Here's how the part is built. I have some questions about the finished solid (model axes, mm). Give positions to 0.01 mm unless a question says otherwise; leave off trailing zeros. Loops run counter-clockwise (first coordinate to the right, second up) from the corner with the lowest first, then second, coordinate; pieces in that order, holes last.
Q1. Suppose I cut it at B-B (z = 43). List the corners of the cut face in (x, y) for me (3 decimals), and give its area (3 significant figures).
Q2. Suppose I cut it at C-C (x = -1). List the corners of the cut face in (y, z) for me.
Q3. I'm going to push flat-ended pins straight in: P1, Ø3, axis at x = 37.5, z = 31.5, coming from the -Y side (3 decimals); P2, Ø1.6, axis at y = -5, z = 55, coming from the +X side (3 decimals); P3, Ø3, axis at x = -16.5, y = -2.5, coming from the +Z side. Where does each tip first touch, or does it pass through?
Q4. Suppose I cut it at A-A (y = -1). List the corners of the cut face in (x, z) for me (3 decimals), and give its area (3 significant figures).
Q5. I need wall thicknesses on probe 1 along X at (y, z) = (-4.5, 82.5) (3 decimals); probe 2 along X at (y, z) = (-1, 75) (3 decimals); probe 3 along Z at (x, y) = (-15, -3). Which ranges of each line are inside material? Lowest first, please.
```python
from build123d import *

# Parameters (mm, degrees)
F1_DEPTH = 6.35
F2_W     = 6.35
F2_H     = 95.25
F3_DEPTH = 3.175


with BuildPart() as f1:
    # F0 (on Front) → F1 (new body)
    with BuildSketch(Plane.XZ):
        with BuildLine():
            Line((-41.275, 0), (0, 0))
            Line((0, 0), (41.275, 0))
            Line((41.275, 0), (41.275, 95.25))
            Line((41.275, 95.25), (22.225, 95.25))
            Line((22.225, 95.25), (22.225, 73.025))
            ThreePointArc((22.225, 73.025), (21.2950640303, 70.7799359697), (19.05, 69.85))
            Line((19.05, 69.85), (-19.05, 69.85))
            ThreePointArc((-19.05, 69.85), (-21.2950640303, 70.7799359697), (-22.225, 73.025))
            Line((-22.225, 73.025), (-22.225, 95.25))
            Line((-22.225, 95.25), (-41.275, 95.25))
            Line((-41.275, 95.25), (-41.275, 0))
        make_face()
    extrude(amount=F1_DEPTH)

    # F2 (on face) → F3 (cut)
    with BuildSketch(Plane.XZ.offset(6.35)):
        with Locations((-38.1, 47.625)):
            Rectangle(F2_W, F2_H)
        with Locations((38.1, 47.625)):
            Rectangle(F2_W, F2_H)
    extrude(amount=-F3_DEPTH, mode=Mode.SUBTRACT)


solid = f1.part
```
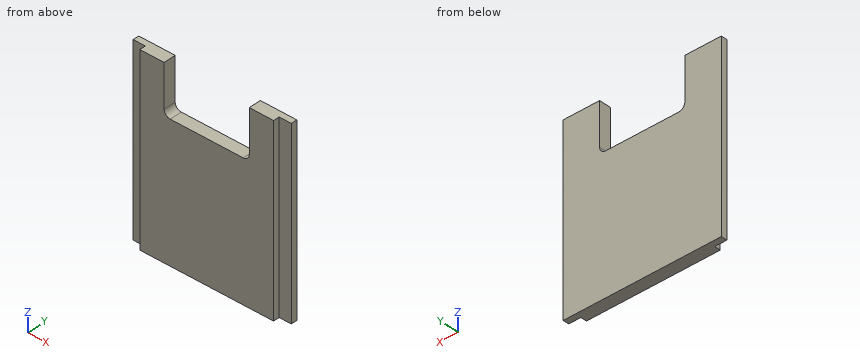
Solutions:
1. outline: (-41.275, -3.175) - (-34.925, -3.175) - (-34.925, -6.35) - (34.925, -6.35) - (34.925, -3.175) - (41.275, -3.175) - (41.275, 0) - (-41.275, 0) - close
1. area: 484 mm2
2. outline: (-6.35, 0) - (0, 0) - (0, 69.85) - (-6.35, 69.85) - close
3. P1: stops at y = -3.175
3. P2: stops at x = 34.925
3. P3: stops at z = 69.85
4. outline: (-41.275, 0) - (41.275, 0) - (41.275, 95.25) - (22.225, 95.25) - (22.225, 73.025) arc R3.175 cw to (19.05, 69.85) - (-19.05, 69.85) arc R3.175 cw to (-22.225, 73.025) - (-22.225, 95.25) - (-41.275, 95.25) - close
4. area: 6,740 mm2
5. probe 1: x = -34.925 to -22.225, 22.225 to 34.925
5. probe 2: x = -41.275 to -22.225, 22.225 to 41.275
5. probe 3: z = 0 to 69.85
